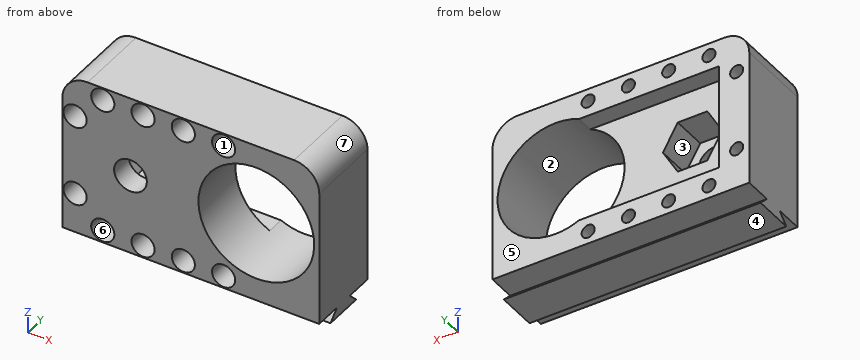
Solid Edge part; units mm, degrees
sketch "Sketch1" plane through (0, 0, 0) normal (0, -1, 0) x (1, 0, 0)
  line L0 (16, 20) -> (-44, 20)
  line L1 (-44, 20) -> (-44, -20)
  line L2 (-44, -20) -> (16, -20)
  line L3 (16, -20) -> (16, 20)
  dimension "D1" = 16
  dimension "D2" = 16
extrude "Protrusion1" add sketch "Sketch1" against normal blind 15
sketch "Sketch2" plane through (-14, 0, 0) normal (0, -1, 0) x (0, 0, -1)
  circle A0 centre (0, 14) radius 11.5
extrude "Cutout1" cut sketch "Sketch2" against normal through all
sketch "Sketch3" plane through (-13.5, 14.5, 0) normal (0, 1, 0) x (0, 0, 1)
  line L0 (-10.5, -19.5) -> (10.5, -19.5)
  line L1 (10.5, -19.5) -> (10.5, 13.5)
  line L2 (10.5, 13.5) -> (-10.5, 13.5)
  line L3 (-10.5, 13.5) -> (-10.5, -19.5)
  dimension "D1" = 10.5
  dimension "D2" = 10.5
extrude "VaciadoExtruido_3" cut sketch "Sketch3" against normal blind 3
hole "Agujero_7" at (-25, 11.5, 0) direction (0, -1, 0) diameter 6.5 end up to next
sketch "Sketch4" plane through (-14, 0, 15) normal (0, -1, 0) x (-1, 0, 0)
  circle A0 centre (8.5, 28.5) radius 1.3
  circle A1 centre (16.5, 28.5) radius 1.3
  circle A2 centre (-7.5, 1.5) radius 1.3
  circle A3 centre (8.5, 1.5) radius 1.3
  circle A4 centre (16.5, 1.5) radius 1.3
  circle A5 centre (22, 23) radius 1.3
  circle A6 centre (22, 7) radius 1.3
  circle A7 centre (0.5, 28.5) radius 1.3
  circle A8 centre (0.5, 1.5) radius 1.3
  circle A9 centre (-7.5, 28.5) radius 1.3
extrude "Cutout2" cut sketch "Sketch4" against normal through all
sketch "Sketch5" plane through (-18.8452, 11.5, 0) normal (0, 1, 0) x (0, 0, -1)
  line L0 (5.1, 9.0993) -> (0, 12.0438)
  line L1 (0, 12.0438) -> (-5.1, 9.0993)
  line L2 (-5.1, 9.0993) -> (-5.1, 3.2103)
  line L3 (-5.1, 3.2103) -> (0, 0.2658)
  line L4 (0, 0.2658) -> (5.1, 3.2103)
  line L5 (5.1, 3.2103) -> (5.1, 9.0993)
extrude "VaciadoExtruido_14" cut sketch "Sketch5" against normal blind 7
sketch "Sketch6" plane through (-14, 0, 0) normal (0, -1, 0) x (-1, 0, 0)
  line L0 (-26.5, -16) -> (24.5, -16)
  line L1 (24.5, -16) -> (24.5, 16)
  line L2 (24.5, 16) -> (-26.5, 16)
  line L3 (-26.5, 16) -> (-26.5, -16)
  line L4 (36.0036, -24.8602) -> (-34.0265, -24.8602)
  line L5 (-34.0265, -24.8602) -> (-34.0265, 20.7723)
  line L6 (-34.0265, 20.7723) -> (36.0036, 20.7723)
  line L7 (36.0036, 20.7723) -> (36.0036, -24.8602)
extrude "Cutout3" cut sketch "Sketch6" against normal through all
sketch "Sketch7" plane through (12.5, 5.75, 0) normal (1, 0, 0) x (0, -1, 0)
  line L0 (-3.75, 16) -> (-5.75, 18)
  line L1 (-5.75, 18) -> (-1.75, 18)
  line L2 (2.25, 18) -> (-1.75, 18)
  line L3 (0.25, 16) -> (2.25, 18)
  line L4 (0.25, 16) -> (-1.75, 16)
  line L5 (-3.75, 16) -> (-1.75, 16)
extrude "ProtrusiónExtruida_10" add sketch "Sketch7" against normal blind 51
fillet "Round1" radius 5 2 edges at (12.5, 7.5, 16) (-38.5, 7.5, 16)
sketch "Sketch8" plane through (-13, 15, 0) normal (0, 1, 0) x (1, 0, 0)
  line L0 (-19.5, 10.5) -> (11, 10.5)
  line L1 (11, 10.5) -> (11, -10.5)
  line L2 (11, -10.5) -> (-19.5, -10.5)
  line L3 (-19.5, -10.5) -> (-19.5, 10.5)
extrude "VaciadoExtruido_31" cut sketch "Sketch8" against normal blind 3
sketch "Sketch9" plane through (-13, 0, 0) normal (0, -1, 0) x (1, 0, 0)
  circle A0 centre (6.5, -13.5) radius 2.3
  circle A1 centre (-1.5, -13.5) radius 2.3
  circle A2 centre (-9.5, -13.5) radius 2.3
  circle A3 centre (-17.5, -13.5) radius 2.3
  circle A4 centre (-23, -8) radius 2.3
  circle A5 centre (-23, 8) radius 2.3
  circle A6 centre (-17.5, 13.5) radius 2.3
  circle A7 centre (-9.5, 13.5) radius 2.3
  circle A8 centre (-1.5, 13.5) radius 2.3
  circle A9 centre (6.5, 13.5) radius 2.3
extrude "Cutout4" cut sketch "Sketch9" against normal blind 8.5
The model under review builds one solid part; all positions refer to its coordinate system, in mm. Face numbers are marked on the shaded views. A direction names the side the tool comes from. Coordinates: 2 decimals unless noted, no trailing zeros. Loops run counter-clockwise (first coordinate to the right, second up) from the corner with the lowest first, then second, coordinate; pieces in that order, holes last. Notation, with made-up numbers: (66, 56) -> (104, 56) arc R14 ccw to (104, 79) -> close; hole circle Ø4 at (64.25, 2.5). An arc over 180 degrees is marked (long way). Answer as CSV lines item,"result".
Item 1: Machinability: for the marked faces 1, 2 and 3, which of the approach directions +Z, -Z, +X, -X, +Y, -Y give a long, thin tool a straight path to every point of the face, cutting with its end or side? Answer none if there is none.
Results below:
face 1,"-Y"
face 2,"+Y, -Y"
face 3,"+Y"
Item 2: For L1, parallel to Z at x = -14.5, y = 12; L2, parallel to X at y = 1.75, z = 13 (3 decimals); L3, parallel to Z at x = 7.5, y = 11, list the stretches that pass through material, from the lowest coordinate up.
Results below:
L1,"z = -16 to -14.8, -12.2 to -10.5, 10.5 to 12.2, 14.8 to 16"
L2,"x = -38.083 to -32.745, -28.255 to -24.745, -20.255 to -16.745, -12.255 to -8.745, -4.255 to 12.083"
L3,"z = -18 to -17.5, -16 to -8.72, 8.72 to 16"
Item 3: Draft analysis for pull direction Z (two halves, no side actions). For the marked faces 4, 5, 6 and 7, state which applies: +Z half, -Z half, draft (parallel to the pull), parting line (faces both ways), or undercut.
Results below:
face 4,"-Z half"
face 5,"draft"
face 6,"undercut"
face 7,"+Z half"
Item 4: Insertion check: pin 1 (3.5 mm diameter, centred on x = -14, z = 13, fed in from -Y); pin 2 (1.4 mm diameter, centred on x = -21.5, z = -13, fed in from -Y); pin 3 (2.5 mm diameter, centred on x = -36, z = 8, fed in from -Y); pin 4 (1.8 mm diameter, centred on x = -12.5, y = 14, fed in from -Z). Each pin has a flat end and moves straight along its axis. Give the tip position at first contact, or say it passes through.
Results below:
pin 1,"stops at y = 0"
pin 2,"stops at y = 8.5"
pin 3,"passes through"
pin 4,"stops at z = -16"
Item 5: Take a section at B-B, the plane x = -14.5. State the section outline as (y, z) points.
Results below:
outline,"(0, -16) -> (5.5, -16) -> (3.5, -18) -> (11.5, -18) -> (9.5, -16) -> (15, -16) -> (15, -14.8) -> (8.5, -14.8) -> (8.5, -15.8) -> (0, -15.8) -> close; (0, -11.2) -> (8.5, -11.2) -> (8.5, -12.2) -> (15, -12.2) -> (15, -10.5) -> (11.5, -10.5) -> (11.5, 10.5) -> (15, 10.5) -> (15, 12.2) -> (8.5, 12.2) -> (8.5, 11.2) -> (0, 11.2) -> close; (0, 15.8) -> (8.5, 15.8) -> (8.5, 14.8) -> (15, 14.8) -> (15, 16) -> (0, 16) -> close"
Item 6: Take a section at A-A, the plane y = 10.25. Count the separate pieces of the cut face and the enclosed holes in it, and give its area (3 significant figures).
Results below:
separate pieces,"2"
enclosed holes,"12"
area,"1,130 mm2"
